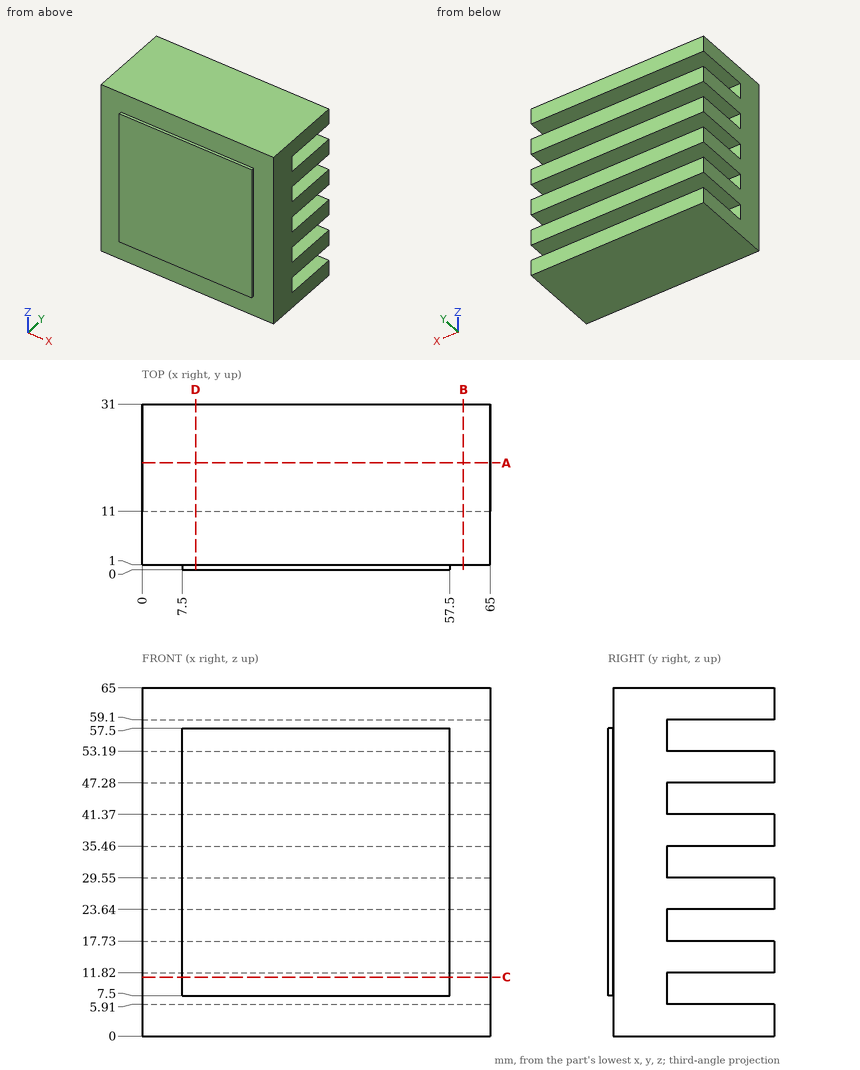
Answer from the drawing. Dimensions are ordinates in mm from the lowest x, y and z of the part. Give positions to 0.01 mm unless a question says otherwise; leave off trailing zeros. Order: outer loops, then holes, each group sorted by start corner. A loop starts at its lowest first (then second) coordinate and runs counter-clockwise, first axis right, second up.
Item 1: Find the intervals of material crossed by probe 1 along Z at (x, y) = (25, 24.5); probe 2 along Y at (x, z) = (22.5, 9.5); probe 3 along Y at (x, z) = (60.5, 55), in increasing order.
From the geometry:
probe 1: z = 0 to 5.91, 11.82 to 17.73, 23.64 to 29.55, 35.46 to 41.37, 47.28 to 53.19, 59.1 to 65
probe 2: y = 0 to 11
probe 3: y = 1 to 11
Item 2: Given pin 1 Ø3 at (x, z) = (19, 20) entering from +Y; pin 2 Ø0.5 at (x, y) = (26, 0.5) entering from -Z, each flat-ended and moving along its own axis, determine where each tip first touches the part or whether it passes through.
From the geometry:
pin 1: stops at y = 11
pin 2: stops at z = 7.5
Item 3: The part is cut by section A-A, the plane y = 20. Give the vertices of the cut face in (x, z), and give its area (3 significant figures).
From the geometry:
outline: (0, 0) - (65, 0) - (65, 5.91) - (0, 5.91) - close; (0, 11.82) - (65, 11.82) - (65, 17.73) - (0, 17.73) - close; (0, 23.64) - (65, 23.64) - (65, 29.55) - (0, 29.55) - close; (0, 35.46) - (65, 35.46) - (65, 41.37) - (0, 41.37) - close; (0, 47.28) - (65, 47.28) - (65, 53.19) - (0, 53.19) - close; (0, 59.1) - (65, 59.1) - (65, 65) - (0, 65) - close
area: 2,300 mm2
Item 4: The part is cut by section D-D, the plane x = 10. Give the vertices of the cut face in (y, z), and give its area (3 significant figures).
From the geometry:
outline: (0, 7.5) - (1, 7.5) - (1, 0) - (31, 0) - (31, 5.91) - (11, 5.91) - (11, 11.82) - (31, 11.82) - (31, 17.73) - (11, 17.73) - (11, 23.64) - (31, 23.64) - (31, 29.55) - (11, 29.55) - (11, 35.46) - (31, 35.46) - (31, 41.37) - (11, 41.37) - (11, 47.28) - (31, 47.28) - (31, 53.19) - (11, 53.19) - (11, 59.1) - (31, 59.1) - (31, 65) - (1, 65) - (1, 57.5) - (0, 57.5) - close
area: 1,410 mm2
Item 5: The part is cut by section B-B, the plane x = 60. Give the vertices of the cut face in (y, z).
From the geometry:
outline: (1, 0) - (31, 0) - (31, 5.91) - (11, 5.91) - (11, 11.82) - (31, 11.82) - (31, 17.73) - (11, 17.73) - (11, 23.64) - (31, 23.64) - (31, 29.55) - (11, 29.55) - (11, 35.46) - (31, 35.46) - (31, 41.37) - (11, 41.37) - (11, 47.28) - (31, 47.28) - (31, 53.19) - (11, 53.19) - (11, 59.1) - (31, 59.1) - (31, 65) - (1, 65) - close
Item 6: The part is cut by section C-C, the plane z = 11. Give the vertices of the cut face in (x, y), and give its area (3 significant figures).
From the geometry:
outline: (0, 1) - (7.5, 1) - (7.5, 0) - (57.5, 0) - (57.5, 1) - (65, 1) - (65, 11) - (0, 11) - close
area: 700 mm2
